The drawing under review shows one solid part. Ordinate dimensions are in mm from its lowest x, y, z. A direction names the side the tool comes from. Coordinates: 2 decimals unless noted, no trailing zeros. Loops run counter-clockwise (first coordinate to the right, second up) from the corner with the lowest first, then second, coordinate; pieces in that order, holes last. Notation, with made-up numbers: (54.5, 35.5) - (78.5, 35.5) arc R20 cw to (78.5, 73.5) - close; hole circle Ø2 at (-7, -27.75). An arc over 180 degrees is marked (long way). Use one line per item in the form item = value. Start each with the question number.
1. Draft analysis for pull direction X (two halves, no side actions). For the marked faces 1, 2 and 3, state which applies: +X half, -X half, draft (parallel to the pull), parting line (faces both ways), or undercut.
2. Add section D-D on y = 4. Give the boundary of the cut face in (x, z).
3. For pin 1 Ø9 at (x, z) = (3, 10) entering from -Y; pin 2 Ø7 at (x, z) = (28, 6.5) entering from -Y; pin 3 Ø12 at (x, z) = (7.5, 15.5) entering from -Y, all flat-tipped, find the tip position at first contact; note any pin that passes through.
4. To check wall thickness, follow probe 1 along X at (y, z) = (7.75, 7.5) (1 decimal); probe 2 along X at (y, z) = (8.05, 18.75); probe 3 along Y at (x, z) = (3, 10.5). State the ranges of each line that lie inside material, in increasing order.
5. Add section C-C on x = 4. Give the boundary of the cut face in (y, z).
6. Add section A-A on z = 18.75. Give the boundary of the cut face in (x, y).
7. Add section B-B on y = 9.25. Give the boundary of the cut face in (x, z).
8. Machinability: for the marked faces 4, 5 and 6, which of the approach directions +Z, -Z, +X, -X, +Y, -Y give a long, thin tool a straight path to every point of the face, cutting with its end or side? Answer none if there is none.
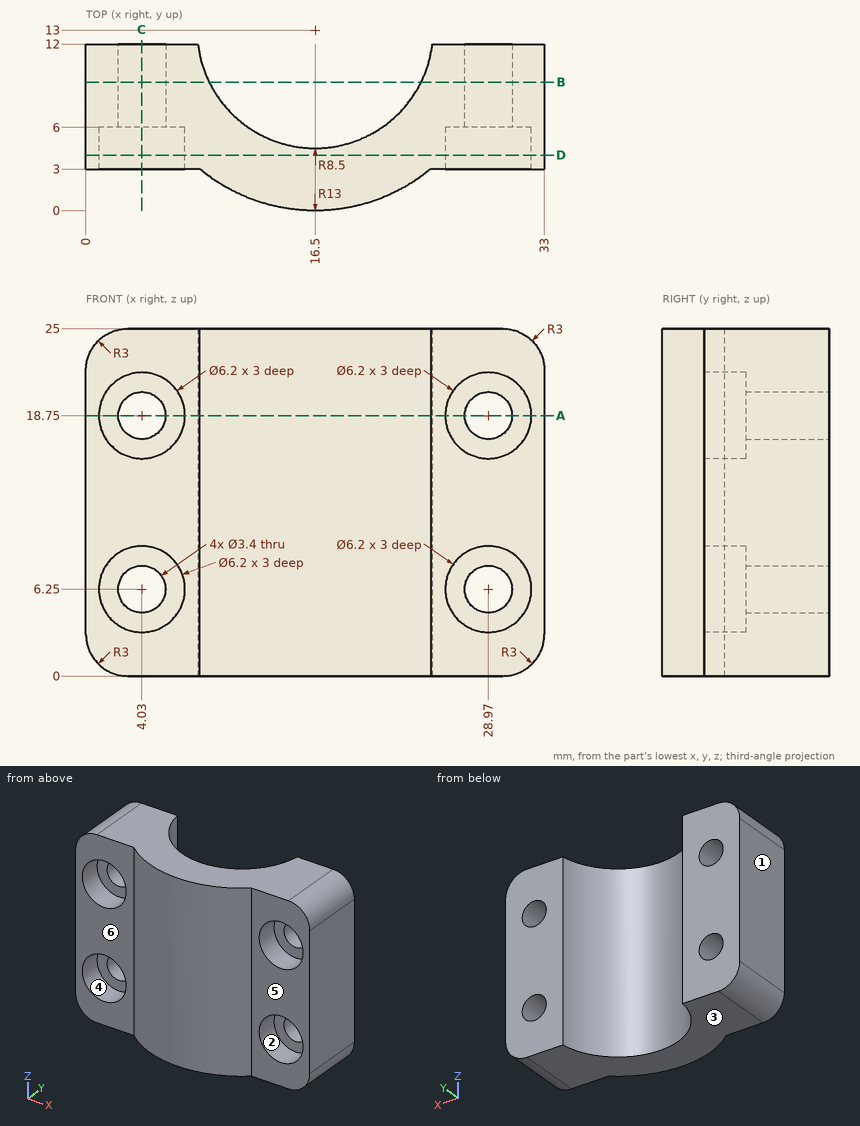
Conclusion:
q1.face_1 = -X half
q1.face_2 = undercut
q1.face_3 = draft
q2.outline = (0, 3) arc R3 ccw to (3, 0) - (30, 0) arc R3 ccw to (33, 3) - (33, 22) arc R3 ccw to (30, 25) - (3, 25) arc R3 ccw to (0, 22) - close; hole circle Ø6.2 at (4.03, 6.25); hole circle Ø6.2 at (4.03, 18.75); hole circle Ø6.2 at (28.97, 6.25); hole circle Ø6.2 at (28.97, 18.75)
q3.pin_1 = 3
q3.pin_2 = 2.75
q3.pin_3 = 0.35
q4.probe_1 = 0 to 2.9, 5.2 to 9.8, 23.2 to 27.8, 30.1 to 33
q4.probe_2 = 0 to 2.33, 5.73 to 9.59, 23.41 to 27.27, 30.67 to 33
q4.probe_3 = 3 to 12
q5.outline = (3, 0) - (12, 0) - (12, 4.55) - (6, 4.55) - (6, 3.15) - (3, 3.15) - close; (3, 9.35) - (6, 9.35) - (6, 7.95) - (12, 7.95) - (12, 17.05) - (6, 17.05) - (6, 15.65) - (3, 15.65) - close; (3, 21.85) - (6, 21.85) - (6, 20.45) - (12, 20.45) - (12, 25) - (3, 25) - close
q6.outline = (0, 3) - (0.93, 3) - (0.93, 6) - (2.33, 6) - (2.33, 12) - (0, 12) - close; (5.73, 6) - (7.13, 6) - (7.13, 3) - (8.19, 3) arc R13 ccw to (24.81, 3) - (25.87, 3) - (25.87, 6) - (27.27, 6) - (27.27, 12) - (24.94, 12) arc R8.5 cw to (8.06, 12) - (5.73, 12) - close; (30.67, 6) - (32.07, 6) - (32.07, 3) - (33, 3) - (33, 12) - (30.67, 12) - close
q7.outline = (0, 3) arc R3 ccw to (3, 0) - (8.87, 0) - (8.87, 25) - (3, 25) arc R3 ccw to (0, 22) - close; (24.13, 0) - (30, 0) arc R3 ccw to (33, 3) - (33, 22) arc R3 ccw to (30, 25) - (24.13, 25) - close; hole circle Ø3.4 at (4.03, 6.25); hole circle Ø3.4 at (4.03, 18.75); hole circle Ø3.4 at (28.97, 6.25); hole circle Ø3.4 at (28.97, 18.75)
q8.face_4 = -Y
q8.face_5 = +Z, -Z, +X, -Y
q8.face_6 = +Z, -Z, -X, -Y
